Read the model definition and answer for the solid it produces. Units are mm, in the model's axes. Face numbers are marked on the shaded views. A direction names the side the tool comes from. Give positions to 0.01 mm unless a question says otherwise; leave off trailing zeros. Order: outer loops, then holes, each group sorted by start corner. A loop starts at its lowest first (then second) coordinate and runs counter-clockwise, first axis right, second up. Notation, with made-up numbers: M -15.5,49.5 L 41.5,49.5 A36 cw 41.5,84.5 Z; hole C -15,77 d5. An arc over 180 degrees is marked long. One line per item, written item: value.
from build123d import *

# Parameters (mm, degrees)
CYLINDER002001_R              = 1.5
CYLINDER002001_DEPTH          = 5
CYLINDER002001_PITCH_ANGLE    = 90
CYLINDER002002_R              = 1.5
CYLINDER002002_DEPTH          = 5
CYLINDER002002_PITCH_ANGLE    = 90
CYLINDER002001001_R           = 1.5
CYLINDER002001001_DEPTH       = 5
CYLINDER002001001_PITCH_ANGLE = 90
CYLINDER_R                    = 1.5
CYLINDER_DEPTH                = 10
CYLINDER002001002_R           = 1.5
CYLINDER002001002_DEPTH       = 10
CYLINDER002001003_R           = 1.5
CYLINDER002001003_DEPTH       = 10
CYLINDER002001002001_R        = 1.5
CYLINDER002001002001_DEPTH    = 10
CYLINDER002_R                 = 1.5
CYLINDER002_DEPTH             = 5
CYLINDER002_PITCH_ANGLE       = 90
BOX003_W                      = 5.5
BOX003_H                      = 2.5
BOX003_DEPTH                  = 5.5
BOX003_PLACEMENT_ANGLE        = -90
BOX004_W                      = 5.5
BOX004_H                      = 2.5
BOX004_DEPTH                  = 5.5
BOX004_PLACEMENT_ANGLE        = -90
BOX005_W                      = 5.5
BOX005_H                      = 2.5
BOX005_DEPTH                  = 5.5
BOX005_PLACEMENT_ANGLE        = -90
BOX006_W                      = 5.5
BOX006_H                      = 2.5
BOX006_DEPTH                  = 5.5
BOX006_ROLL_ANGLE             = 90
BOX007_W                      = 5.5
BOX007_H                      = 2.5
BOX007_DEPTH                  = 5.5
BOX007_ROLL_ANGLE             = 90
BOX006001_W                   = 5.5
BOX006001_H                   = 2.5
BOX006001_DEPTH               = 5.5
BOX006001_ROLL_ANGLE          = 90
BOX007001_W                   = 5.5
BOX007001_H                   = 2.5
BOX007001_DEPTH               = 5.5
BOX007001_ROLL_ANGLE          = 90
BOX002_W                      = 5.5
BOX002_H                      = 2.5
BOX002_DEPTH                  = 5.5
BOX002_PLACEMENT_ANGLE        = -90
BOX001_W                      = 66.199997
BOX001_H                      = 66.199997
BOX001_DEPTH                  = 10
BOX_W                         = 76.199997
BOX_H                         = 96.199997
BOX_DEPTH                     = 10


with BuildPart() as cylinder002001:
    # Cylinder002001 → Cylinder002001 (new body)
    with BuildSketch(Plane.XY):
        Circle(CYLINDER002001_R)
    extrude(amount=CYLINDER002001_DEPTH)


with BuildPart() as cylinder002001_1:
    # Cylinder002001 pitch: moved
    add(cylinder002001.part.rotate(Axis((0, 0, 0), (0, 1, 0)), CYLINDER002001_PITCH_ANGLE))


with BuildPart() as cylinder002001_2:
    # Cylinder002001 placement: moved
    add(cylinder002001_1.part.moved(Location((71.2, 35.4, 5))))


with BuildPart() as cylinder002002:
    # Cylinder002002 → Cylinder002002 (new body)
    with BuildSketch(Plane.XY):
        Circle(CYLINDER002002_R)
    extrude(amount=CYLINDER002002_DEPTH)


with BuildPart() as cylinder002002_1:
    # Cylinder002002 pitch: moved
    add(cylinder002002.part.rotate(Axis((0, 0, 0), (0, 1, 0)), CYLINDER002002_PITCH_ANGLE))


with BuildPart() as cylinder002002_2:
    # Cylinder002002 placement: moved
    add(cylinder002002_1.part.moved(Location((-0.8, 60.8, 5))))


with BuildPart() as cylinder002001001:
    # Cylinder002001001 → Cylinder002001001 (new body)
    with BuildSketch(Plane.XY):
        Circle(CYLINDER002001001_R)
    extrude(amount=CYLINDER002001001_DEPTH)


with BuildPart() as cylinder002001001_1:
    # Cylinder002001001 pitch: moved
    add(cylinder002001001.part.rotate(Axis((0, 0, 0), (0, 1, 0)), CYLINDER002001001_PITCH_ANGLE))


with BuildPart() as cylinder002001001_2:
    # Cylinder002001001 placement: moved
    add(cylinder002001001_1.part.moved(Location((-0.8, 35.4, 5))))


with BuildPart() as cylinder:
    # Cylinder → Cylinder (new body)
    with BuildSketch(Plane(origin=(25.4, 5, 0), x_dir=(1, 0, 0), z_dir=(0, 0, 1))):
        Circle(CYLINDER_R)
    extrude(amount=CYLINDER_DEPTH)


with BuildPart() as cylinder002001002:
    # Cylinder002001002 → Cylinder002001002 (new body)
    with BuildSketch(Plane(origin=(50.8, 5, 0), x_dir=(1, 0, 0), z_dir=(0, 0, 1))):
        Circle(CYLINDER002001002_R)
    extrude(amount=CYLINDER002001002_DEPTH)


with BuildPart() as cylinder002001003:
    # Cylinder002001003 → Cylinder002001003 (new body)
    with BuildSketch(Plane(origin=(25.4, 91.2, 0), x_dir=(1, 0, 0), z_dir=(0, 0, 1))):
        Circle(CYLINDER002001003_R)
    extrude(amount=CYLINDER002001003_DEPTH)


with BuildPart() as cylinder002001002001:
    # Cylinder002001002001 → Cylinder002001002001 (new body)
    with BuildSketch(Plane(origin=(50.8, 91.2, 0), x_dir=(1, 0, 0), z_dir=(0, 0, 1))):
        Circle(CYLINDER002001002001_R)
    extrude(amount=CYLINDER002001002001_DEPTH)


with BuildPart() as cylinder002:
    # Cylinder002 → Cylinder002 (new body)
    with BuildSketch(Plane.XY):
        Circle(CYLINDER002_R)
    extrude(amount=CYLINDER002_DEPTH)


with BuildPart() as cylinder002_1:
    # Cylinder002 pitch: moved
    add(cylinder002.part.rotate(Axis((0, 0, 0), (0, 1, 0)), CYLINDER002_PITCH_ANGLE))


with BuildPart() as cylinder002_2:
    # Cylinder002 placement: moved
    add(cylinder002_1.part.moved(Location((71.2, 60.8, 5))))


with BuildPart() as box003:
    # Box003 → Box003 (new body)
    with BuildSketch(Plane.XY):
        with Locations((2.75, 1.25)):
            Rectangle(BOX003_W, BOX003_H)
    extrude(amount=BOX003_DEPTH)


with BuildPart() as box003_1:
    # Box003 placement: moved
    add(box003.part.moved(Location((71.19, 63.55, 2.5))).rotate(Axis((71.19, 63.55, 2.5), (0, 0, 1)), BOX003_PLACEMENT_ANGLE))


with BuildPart() as box004:
    # Box004 → Box004 (new body)
    with BuildSketch(Plane.XY):
        with Locations((2.75, 1.25)):
            Rectangle(BOX004_W, BOX004_H)
    extrude(amount=BOX004_DEPTH)


with BuildPart() as box004_1:
    # Box004 placement: moved
    add(box004.part.moved(Location((2.5, 63.55, 2.5))).rotate(Axis((2.5, 63.55, 2.5), (0, 0, 1)), BOX004_PLACEMENT_ANGLE))


with BuildPart() as box005:
    # Box005 → Box005 (new body)
    with BuildSketch(Plane.XY):
        with Locations((2.75, 1.25)):
            Rectangle(BOX005_W, BOX005_H)
    extrude(amount=BOX005_DEPTH)


with BuildPart() as box005_1:
    # Box005 placement: moved
    add(box005.part.moved(Location((2.5, 38.15, 2.5))).rotate(Axis((2.5, 38.15, 2.5), (0, 0, 1)), BOX005_PLACEMENT_ANGLE))


with BuildPart() as box006:
    # Box006 → Box006 (new body)
    with BuildSketch(Plane.XY):
        with Locations((2.75, 1.25)):
            Rectangle(BOX006_W, BOX006_H)
    extrude(amount=BOX006_DEPTH)


with BuildPart() as box006_1:
    # Box006 roll: moved
    add(box006.part.rotate(Axis((0, 0, 0), (1, 0, 0)), BOX006_ROLL_ANGLE))


with BuildPart() as box006_2:
    # Box006 placement: moved
    add(box006_1.part.moved(Location((22.65, 7.75, 7.5))))


with BuildPart() as box007:
    # Box007 → Box007 (new body)
    with BuildSketch(Plane.XY):
        with Locations((2.75, 1.25)):
            Rectangle(BOX007_W, BOX007_H)
    extrude(amount=BOX007_DEPTH)


with BuildPart() as box007_1:
    # Box007 roll: moved
    add(box007.part.rotate(Axis((0, 0, 0), (1, 0, 0)), BOX007_ROLL_ANGLE))


with BuildPart() as box007_2:
    # Box007 placement: moved
    add(box007_1.part.moved(Location((48.05, 7.75, 7.5))))


with BuildPart() as box006001:
    # Box006001 → Box006001 (new body)
    with BuildSketch(Plane.XY):
        with Locations((2.75, 1.25)):
            Rectangle(BOX006001_W, BOX006001_H)
    extrude(amount=BOX006001_DEPTH)


with BuildPart() as box006001_1:
    # Box006001 roll: moved
    add(box006001.part.rotate(Axis((0, 0, 0), (1, 0, 0)), BOX006001_ROLL_ANGLE))


with BuildPart() as box006001_2:
    # Box006001 placement: moved
    add(box006001_1.part.moved(Location((22.65, 93.95, 7.5))))


with BuildPart() as box007001:
    # Box007001 → Box007001 (new body)
    with BuildSketch(Plane.XY):
        with Locations((2.75, 1.25)):
            Rectangle(BOX007001_W, BOX007001_H)
    extrude(amount=BOX007001_DEPTH)


with BuildPart() as box007001_1:
    # Box007001 roll: moved
    add(box007001.part.rotate(Axis((0, 0, 0), (1, 0, 0)), BOX007001_ROLL_ANGLE))


with BuildPart() as box007001_2:
    # Box007001 placement: moved
    add(box007001_1.part.moved(Location((48.05, 93.95, 7.5))))


with BuildPart() as box002:
    # Box002 → Box002 (new body)
    with BuildSketch(Plane.XY):
        with Locations((2.75, 1.25)):
            Rectangle(BOX002_W, BOX002_H)
    extrude(amount=BOX002_DEPTH)


with BuildPart() as box002_1:
    # Box002 placement: moved
    add(box002.part.moved(Location((71.19, 38.15, 2.5))).rotate(Axis((71.19, 38.15, 2.5), (0, 0, 1)), BOX002_PLACEMENT_ANGLE))


with BuildPart() as box001:
    # Box001 → Box001 (new body)
    with BuildSketch(Plane(origin=(5, 15, 0), x_dir=(1, 0, 0), z_dir=(0, 0, 1))):
        with Locations((33.099998, 33.099998)):
            Rectangle(BOX001_W, BOX001_H)
    extrude(amount=BOX001_DEPTH)


with BuildPart() as cut016:
    # Box → Box (new body)
    with BuildSketch(Plane.XY):
        with Locations((38.099998, 48.099998)):
            Rectangle(BOX_W, BOX_H)
    extrude(amount=BOX_DEPTH)

    # Cut: cut Box001
    add(box001.part, mode=Mode.SUBTRACT)

    # Cut001: cut Box002
    add(box002_1.part, mode=Mode.SUBTRACT)

    # Cut002: cut Box007001
    add(box007001_2.part, mode=Mode.SUBTRACT)

    # Cut003: cut Box006001
    add(box006001_2.part, mode=Mode.SUBTRACT)

    # Cut004: cut Box007
    add(box007_2.part, mode=Mode.SUBTRACT)

    # Cut005: cut Box006
    add(box006_2.part, mode=Mode.SUBTRACT)

    # Cut006: cut Box005
    add(box005_1.part, mode=Mode.SUBTRACT)

    # Cut007: cut Box004
    add(box004_1.part, mode=Mode.SUBTRACT)

    # Cut008: cut Box003
    add(box003_1.part, mode=Mode.SUBTRACT)

    # Cut009: cut Cylinder002
    add(cylinder002_2.part, mode=Mode.SUBTRACT)

    # Cut010: cut Cylinder002001002001
    add(cylinder002001002001.part, mode=Mode.SUBTRACT)

    # Cut011: cut Cylinder002001003
    add(cylinder002001003.part, mode=Mode.SUBTRACT)

    # Cut012: cut Cylinder002001002
    add(cylinder002001002.part, mode=Mode.SUBTRACT)

    # Cut013: cut Cylinder
    add(cylinder.part, mode=Mode.SUBTRACT)

    # Cut014: cut Cylinder002001001
    add(cylinder002001001_2.part, mode=Mode.SUBTRACT)

    # Cut015: cut Cylinder002002
    add(cylinder002002_2.part, mode=Mode.SUBTRACT)

    # Cut016: cut Cylinder002001
    add(cylinder002001_2.part, mode=Mode.SUBTRACT)


solid = cut016.part
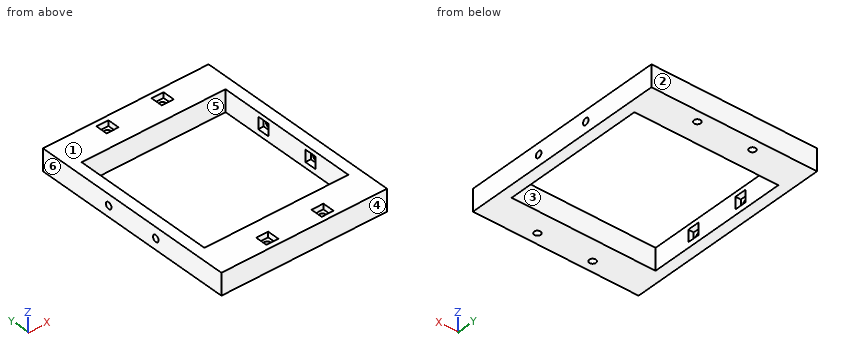
1) Find section A-A, the plane y = 5. Write down the section's boundary in (x, z).
Reported:
outline: M 0,0 L 23.9,0 L 23.9,7.5 L 22.65,7.5 L 22.65,10 L 0,10 Z; M 26.9,0 L 49.3,0 L 49.3,7.5 L 48.05,7.5 L 48.05,10 L 28.15,10 L 28.15,7.5 L 26.9,7.5 Z; M 52.3,0 L 76.2,0 L 76.2,10 L 53.55,10 L 53.55,7.5 L 52.3,7.5 Z
2) Find section C-C, the plane x = 40. Write down the section's boundary in (y, z).
Reported:
outline: M 0,0 L 15,0 L 15,10 L 0,10 Z; M 81.2,0 L 96.2,0 L 96.2,10 L 81.2,10 Z
3) Determine the mould class of the marked faces 1, 2, 3 and 4 for opening direction Y: +Y half, -Y half, draft (parallel to the pull), parting line (faces both ways), or undercut.
Reported:
face 1: draft
face 2: +Y half
face 3: undercut
face 4: -Y half
4) Which of the six approach directions +Z, -Z, +X, -X, +Y, -Y give full straight-line access (tool end or side, diameter ignored) to the marked faces 5 and 6?
Reported:
face 5: +Z, -Z
face 6: +Z, -Z, -X, +Y, -Y
5) Consider probe 1 along X at (y, z) = (91.2, 5.5); probe 2 along Y at (x, z) = (25.4, 4.5); probe 3 along Y at (x, z) = (75.3, 5). Determine where each line is inside the solid, lowest interval first.
Reported:
probe 1: x = 0 to 23.9, 26.9 to 49.3, 52.3 to 76.2
probe 2: y = 0 to 3.5, 6.5 to 15, 81.2 to 89.7, 92.7 to 96.2
probe 3: y = 0 to 33.9, 36.9 to 59.3, 62.3 to 96.2
6) Find section D-D, the plane y = 48. Write down the section's boundary in (x, z), plus the area to 3 significant figures.
Reported:
outline: M 0,0 L 5,0 L 5,10 L 0,10 Z; M 71.2,0 L 76.2,0 L 76.2,10 L 71.2,10 Z
area: 100 mm^2
7) Each of these flat-tipped pins is pushed along its axis until it touches: pin 1 Ø8 at (x, y) = (12, 61.5) entering from -Z; pin 2 Ø4 at (x, y) = (25.4, 5) entering from +Z. Where does it stop, or does it pass through?
Reported:
pin 1: passes through
pin 2: stops at z = 7.5
8) Find section B-B, the plane z = 1.5. Write down the section's boundary in (x, y).
Reported:
outline: M 0,0 L 76.2,0 L 76.2,96.2 L 0,96.2 Z; hole M 5,15 L 71.2,15 L 71.2,81.2 L 5,81.2 Z; hole C 25.4,5 d3; hole C 25.4,91.2 d3; hole C 50.8,5 d3; hole C 50.8,91.2 d3
